Design review of the part shown in the three views and the two pictorial views. Dimensions are in mm from the part's minimum x, y and z. A direction names the side the tool comes from. Coordinates: 2 decimals unless noted, no trailing zeros. Loops run counter-clockwise (first coordinate to the right, second up) from the corner with the lowest first, then second, coordinate; pieces in that order, holes last. Notation, with made-up numbers: (-7, 59) -> (45, 59) arc R15 ccw to (45, 86) -> close; hole circle Ø4 at (-12, 66). An arc over 180 degrees is marked (long way). One line per item, written item: value. Start each with the question number.
1. Machinability: for the marked faces 5 and 6, which of the approach directions +Z, -Z, +X, -X, +Y, -Y give a long, thin tool a straight path to every point of the face, cutting with its end or side? Answer none if there is none.
2. Add section B-B on x = 59. Write out the cut boundary in (y, z).
3. Add section D-D on y = 43. Write out the cut boundary in (x, z), plus the area to 3 significant figures.
4. Draft analysis for pull direction X (two halves, no side actions). For the marked faces 1, 2, 3 and 4, state which applies: pulls with the +X half, pulls with the -X half, needs draft (parallel to the pull), parting line crosses it, or undercut.
5. Add section C-C on x = 77. Write out the cut boundary in (y, z).
6. Insertion check: pin 1 (2 mm diameter, centred on y = 28, z = 28.5, fed in from -X) (1 decimal). The pin has a flat end and moves straight along its axis. Give the tip position at first contact, or say it passes through.
7. For probe 1 along Y at (x, z) = (71.5, 37.5); probe 2 along X at (y, z) = (18, 37); probe 3 along Z at (x, y) = (41.5, 65.5), list the stretches that pass through material, from the lowest coordinate up.
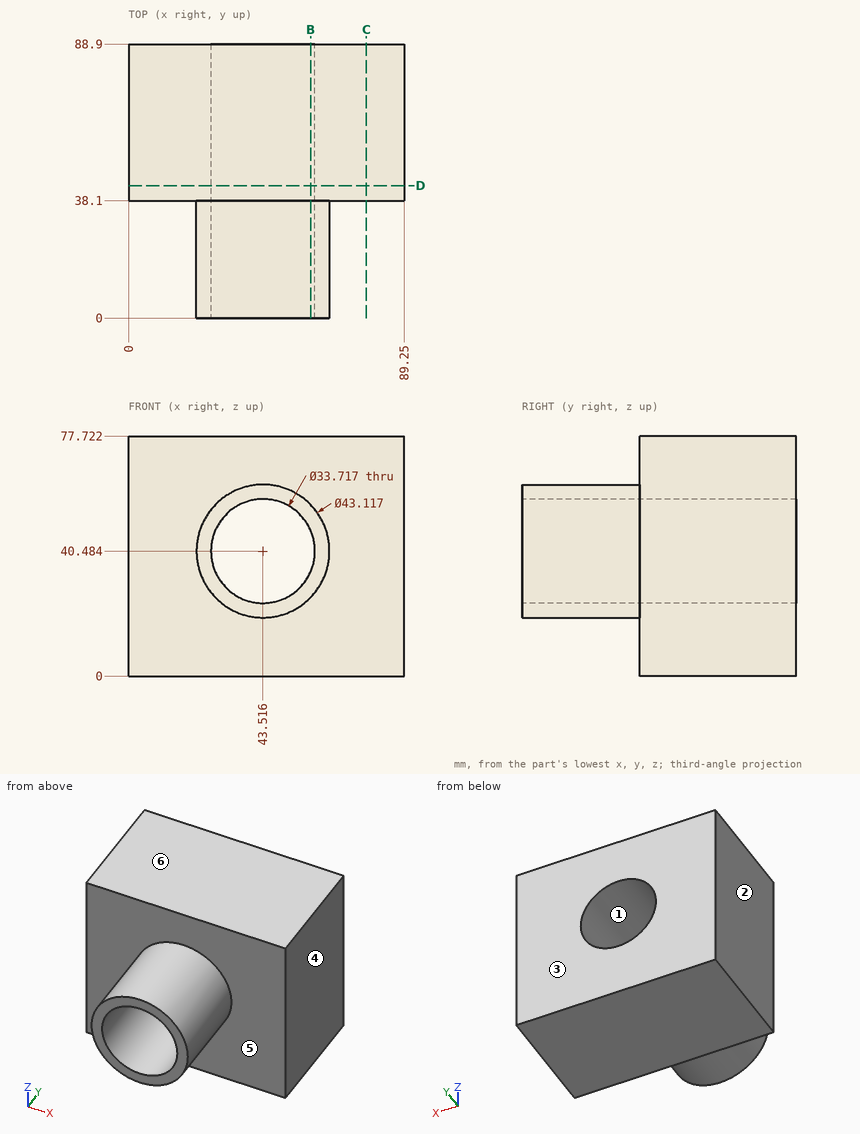
Worked answers:
1. face 5: -Y
1. face 6: +Z, +X, -X, +Y, -Y
2. outline: (0, 25.48) -> (38.1, 25.48) -> (38.1, 0) -> (88.9, 0) -> (88.9, 33.82) -> (0, 33.82) -> close; (0, 47.15) -> (88.9, 47.15) -> (88.9, 77.72) -> (38.1, 77.72) -> (38.1, 55.48) -> (0, 55.48) -> close
3. outline: (0, 0) -> (89.25, 0) -> (89.25, 77.72) -> (0, 77.72) -> close; hole circle Ø33.72 at (43.52, 40.48)
3. area: 6,040 mm²
4. face 1: undercut
4. face 2: pulls with the -X half
4. face 3: needs draft
4. face 4: pulls with the +X half
5. outline: (38.1, 0) -> (88.9, 0) -> (88.9, 77.72) -> (38.1, 77.72) -> close
6. pin 1: stops at x = 25
7. probe 1: y = 38.1 to 88.9
7. probe 2: x = 22.24 to 27.02, 60.01 to 64.79
7. probe 3: z = 0 to 23.75, 57.22 to 77.72
